```python
from build123d import *

# Parameters (mm, degrees)
F0_R          = 4.7625
F1_DEPTH      = 9.525
F1_DEPTH_BACK = 6.35
F3_DEPTH      = 9.526
F4_R          = 15.24
F5_DEPTH      = 7.75
F6_R          = 2.6035
F7_DEPTH      = 13.97
F8_SIZE       = 1.5
F9_SIZE       = 3
F10_S5_R      = 2.6035
F10_T6_DEPTH  = 14
F10_S7_R      = 2.6035
F10_T8_DEPTH  = 14
F10_S9_R      = 2.6035
F10_T10_DEPTH = 14


# Not quite as in the source:
# - a fillet or chamfer that OpenCascade refuses, or shapes differently, is made with other operations: its cross-section is extruded or revolved along the edge and cut away or added


with BuildPart() as f1:
    # F0 (on Top) → F1 (new body, two sides)
    with BuildSketch(Plane.XY) as f1_sk:
        Circle(F0_R)
    extrude(amount=F1_DEPTH)
    extrude(f1_sk.sketch, amount=-F1_DEPTH_BACK)

    # F2 (on Top) → F3 (cut, through all)
    with BuildSketch(Plane.XY):
        with BuildLine():
            ThreePointArc((1.9843134833, -2.25), (2.7343134833, -1.2343134833), (3, 0))
            ThreePointArc((3, 0), (2.7343134833, 1.2343134833), (1.9843134833, 2.25))
            Line((1.9843134833, 2.25), (-1.9843134833, 2.25))
            ThreePointArc((-1.9843134833, 2.25), (-3, 0), (-1.9843134833, -2.25))
            Line((-1.9843134833, -2.25), (1.9843134833, -2.25))
        make_face()
    extrude(amount=F3_DEPTH, mode=Mode.SUBTRACT)

    # F4 (on Top) → F5 (join)
    with BuildSketch(Plane.XY):
        Circle(F4_R)
    extrude(amount=-F5_DEPTH)

    # F6 (on face) → F7 (cut)
    with BuildSketch(Plane(origin=(0, 0, -7.75), x_dir=(1, 0, 0), z_dir=(0, 0, -1))):
        with Locations((1.0674559099, -7.8653953575)):
            Circle(F6_R)
        with Locations((6.2779042355, 4.8571416142)):
            Circle(F6_R)
        with Locations((-7.3453601454, 3.0082537434)):
            Circle(F6_R)
    extrude(amount=-F7_DEPTH, mode=Mode.SUBTRACT)

    # F8
    f8_edges = [f1.edges().sort_by_distance(p)[0] for p in [
        (-15.24, 0, -7.75),
    ]]
    chamfer(f8_edges, length=F8_SIZE)

    # F9
    f9_edges = [f1.edges().sort_by_distance(p)[0] for p in [
        (-15.24, 0, 0),
    ]]
    chamfer(f9_edges, length=F9_SIZE)

    # F10: fillet of radius 3.175 on 1 edges, made by hand


with BuildPart() as f10_tool2:
    # F10_s3 → F10_t4 (revolve)
    with BuildSketch(Plane.XZ):
        with BuildLine():
            ThreePointArc((7.9375, 0), (5.6924359697, 0.9299359697), (4.7625, 3.175))
            Line((4.7625, 3.175), (4.7625, 0))
            Line((4.7625, 0), (7.9375, 0))
        make_face()
    revolve(axis=Axis((0, 0, 0), (0, 0, 1)))

    # F10_s5 → F10_t6 (cut, symmetric)
    with BuildSketch(Plane.XY.offset(2.7)):
        with Locations((-7.3453601454, -3.0082537434)):
            Circle(F10_S5_R)
    extrude(amount=F10_T6_DEPTH, both=True, mode=Mode.SUBTRACT)

    # F10_s7 → F10_t8 (cut, symmetric)
    with BuildSketch(Plane.XY.offset(2.7)):
        with Locations((6.2779042355, -4.8571416142)):
            Circle(F10_S7_R)
    extrude(amount=F10_T8_DEPTH, both=True, mode=Mode.SUBTRACT)

    # F10_s9 → F10_t10 (cut, symmetric)
    with BuildSketch(Plane.XY.offset(2.7)):
        with Locations((1.0674559099, 7.8653953575)):
            Circle(F10_S9_R)
    extrude(amount=F10_T10_DEPTH, both=True, mode=Mode.SUBTRACT)


with BuildPart() as f1_1:
    add(f1.part)

    # F10_t1: union F10_tool2
    add(f10_tool2.part)


solid = f1_1.part
```
For this review, take the finished solid that the model builds, in its own axes (mm). A direction names the side the tool comes from. Give positions to 0.01 mm unless a question says otherwise; leave off trailing zeros. Write each loop counter-clockwise with the first axis right and the second up, starting at its lowest first coordinate (ties: lowest second). Pieces come first, ordered by that corner, then holes. Notation, with made-up numbers: M 6,-21 L 36,-21 A22 cw 36,6 Z; hole C -10,12 d6. An arc over 180 degrees is marked long. Answer as CSV lines item,"result".
1. For pin 1 (4.5 mm diameter, centred on x = -1, z = 6.5, fed in from +Y); pin 2 (3 mm diameter, centred on y = 5.5, z = -5.5, fed in from +X); pin 3 (3.5 mm diameter, centred on x = 1, y = 0, fed in from +Z), all flat-tipped, find the tip position at first contact; note any pin that passes through.
Findings:
pin 1,"stops at y = 4.76"
pin 2,"stops at x = 14.71"
pin 3,"stops at z = 0"
2. Consider section C-C, the plane z = 2.75. Write out the cut boundary in (x, y), then the cut area to 3 significant figures.
Findings:
outline,"C 0,0 d9.58; hole M -1.98,-2.25 L 1.98,-2.25 A3 ccw 1.98,2.25 L -1.98,2.25 A3 ccw Z"
area,"47.9 mm2"
3. Wall thickness on line 1 (Z direction, x = 6.5, y = 7); line 2 (Y direction, x = -8, z = -4.75); line 3 (Y direction, x = 4, z = -6.5): over which ranges is each line inside the solid? List them lowest first.
Findings:
line 1,"z = -7.75 to 0"
line 2,"y = -12.97 to -5.53, -0.49 to 12.97"
line 3,"y = -14.45 to -6.12, -3.6 to 14.45"
4. For faces 1 (the cylindrical face through (-3, 0, 5)), 2 (the flat face through (0, -3, 9.525)), list the 3-axis set-ups (+Z, -Z, +X, -X, +Y, -Y) from which the entire face can be reached by the end or side of a thin tool; tool diameter is ignored.
Findings:
face 1,"+Z"
face 2,"+Z, +X, -X, +Y, -Y"
5. Consider section D-D, the plane z = -2.5. Write out the cut boundary in (x, y).
Findings:
outline,"C 0,0 d29.48; hole C -7.35,-3.01 d5.21; hole C 1.07,7.87 d5.21; hole C 6.28,-4.86 d5.21"
